CAD build for the part. Positions are in the model's coordinates, mm. Face numbers are marked on the shaded views. Give positions to 0.01 mm unless a question says otherwise; leave off trailing zeros.
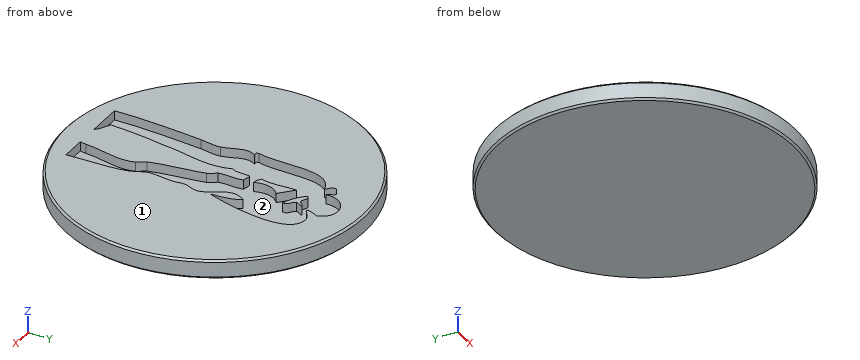
from build123d import *

# Parameters (mm, degrees)
POCKET_DEPTH = 1.25


with BuildPart() as part:
    # Sketch (on DatumPlane) → Revolution (revolve)
    with BuildSketch(Plane.YZ):
        Polygon((0, 0), (0, -2.5), (19.75, -2.5), (20, -2.25), (20, -0.25), (19.75, 0), align=None)
    revolve(axis=Axis((0, 0, 0), (0, 0, 1)))

    # Sketch005 (on DatumPlane) → Pocket (cut)
    with BuildSketch(Plane.XY):
        with BuildLine():
            add(Edge.make_bspline(
                [(2.212734, -16.79531), (2.353913, -15.955428)],
                knots=[0, 0, 11.60658, 11.60658], degree=1))
            add(Edge.make_bspline(
                [(2.353913, -15.955428), (2.452386, -13.484431), (3.666422, -11.326317), (2.913712, -8.958563)],
                knots=[0, 0, 0, 0, 1, 1, 1, 1], degree=3))
            add(Edge.make_bspline(
                [(2.913712, -8.958563), (2.776863, -8.528936), (2.33689, -8.25553), (2.213762, -7.839185)],
                knots=[0, 0, 0, 0, 1, 1, 1, 1], degree=3))
            add(Edge.make_bspline(
                [(2.213762, -7.839185), (1.63261, -5.878384), (1.420254, -2.638828), (0.954306, -0.562751)],
                knots=[0, 0, 0, 0, 1, 1, 1, 1], degree=3))
            add(Edge.make_bspline(
                [(0.954306, -0.562751), (0.837488, -0.042136), (0.287742, 0.418016), (0.254795, 0.556627)],
                knots=[0, 0, 0, 0, 1, 1, 1, 1], degree=3))
            add(Edge.make_bspline(
                [(0.254795, 0.556627), (0.035836, 1.475243), (0.405146, 2.931279), (0.114644, 3.915201)],
                knots=[0, 0, 0, 0, 1, 1, 1, 1], degree=3))
            add(Edge.make_bspline(
                [(0.114644, 3.915201), (-0.335749, 3.884236), (-0.477001, 4.162705), (-1.004588, 4.055279)],
                knots=[0, 0, 0, 0, 1, 1, 1, 1], degree=3))
            add(Edge.make_bspline(
                [(-1.004588, 4.055279), (-1.121992, 3.360832), (-0.906555, 2.162059), (-1.424455, 1.536367)],
                knots=[0, 0, 0, 0, 1, 1, 1, 1], degree=3))
            add(Edge.make_bspline(
                [(-1.424455, 1.536367), (-0.190168, -1.482321), (-1.911464, -5.34911), (-1.969652, -7.903684)],
                knots=[0, 0, 0, 0, 1, 1, 1, 1], degree=3))
            add(Edge.make_bspline(
                [(-1.969652, -7.903684), (-2.432446, -10.377469), (-2.703357, -13.113506), (-2.823623, -15.53644)],
                knots=[0, 0, 0, 0, 1, 1, 1, 1], degree=3))
            add(Edge.make_bspline(
                [(-2.823623, -15.53644), (-2.274023, -16.012809), (-1.385932, -16.150099), (-1.004588, -16.795897)],
                knots=[0, 0, 0, 0, 1, 1, 1, 1], degree=3))
            add(Edge.make_bspline(
                [(-1.004588, -16.795897), (-5.762036, -16.795897)],
                knots=[0, 0, 64.835, 64.835], degree=1))
            add(Edge.make_bspline(
                [(-5.762036, -16.795897), (-5.908571, -13.463225), (-5.538601, -8.73975), (-5.202677, -4.901359)],
                knots=[0, 0, 0, 0, 1, 1, 1, 1], degree=3))
            add(Edge.make_bspline(
                [(-5.202677, -4.901359), (-5.116898, -3.924994), (-4.784204, -3.058916), (-4.922814, -2.102804)],
                knots=[0, 0, 0, 0, 1, 1, 1, 1], degree=3))
            add(Edge.make_bspline(
                [(-4.922814, -2.102804), (-5.15799, -0.475138), (-6.392498, 0.658255), (-5.342242, 2.235731)],
                knots=[0, 0, 0, 0, 1, 1, 1, 1], degree=3))
            add(Edge.make_bspline(
                [(-5.342242, 2.235731), (-5.698637, 2.163087), (-5.885237, 1.997106), (-5.902261, 2.515373)],
                knots=[0, 0, 0, 0, 1, 1, 1, 1], degree=3))
            add(Edge.make_bspline(
                [(-5.902261, 2.515373), (-4.959136, 5.955324), (-6.879579, 11.869573), (-2.963554, 13.011331)],
                knots=[0, 0, 0, 0, 1, 1, 1, 1], degree=3))
            add(Edge.make_bspline(
                [(-2.963554, 13.011331), (-2.683178, 13.346374), (-3.817451, 13.457541), (-3.523427, 14.270347)],
                knots=[0, 0, 0, 0, 1, 1, 1, 1], degree=3))
            add(Edge.make_bspline(
                [(-3.523427, 14.270347), (-3.140321, 14.400739), (-2.926572, 14.699607), (-2.543613, 14.830292)],
                knots=[0, 0, 0, 0, 1, 1, 1, 1], degree=3))
            add(Edge.make_bspline(
                [(-2.543613, 14.830292), (-2.053816, 14.76051), (-2.204608, 14.0497), (-1.844029, 13.850773)],
                knots=[0, 0, 0, 0, 1, 1, 1, 1], degree=3))
            add(Edge.make_bspline(
                [(-1.844029, 13.850773), (-2.144071, 17.003889), (1.974624, 18.085918), (2.773854, 15.250087)],
                knots=[0, 0, 0, 0, 1, 1, 1, 1], degree=3))
            add(Edge.make_bspline(
                [(2.773854, 15.250087), (2.592685, 14.684491), (2.246708, 14.284215), (2.213762, 13.570469)],
                knots=[0, 0, 0, 0, 1, 1, 1, 1], degree=3))
            add(Edge.make_bspline(
                [(2.213762, 13.570469), (2.792786, 13.662925), (3.280014, 14.548962), (4.172728, 14.550283)],
                knots=[0, 0, 0, 0, 1, 1, 1, 1], degree=3))
            add(Edge.make_bspline(
                [(4.172728, 14.550283), (8.655083, 14.556593), (5.532639, 4.064598), (4.732674, 2.096606)],
                knots=[0, 0, 0, 0, 1, 1, 1, 1], degree=3))
            add(Edge.make_bspline(
                [(4.732674, 2.096606), (4.690702, 3.640108), (4.551504, 5.086751), (3.893159, 6.014246)],
                knots=[0, 0, 0, 0, 1, 1, 1, 1], degree=3))
            add(Edge.make_bspline(
                [(3.893159, 6.014246), (2.13422, 3.558659), (4.761805, 2.306173), (4.872605, 0.416989)],
                knots=[0, 0, 0, 0, 1, 1, 1, 1], degree=3))
            add(Edge.make_bspline(
                [(4.872605, 0.416989), (4.917146, -0.345406), (4.402694, -0.841587), (4.312953, -1.541977)],
                knots=[0, 0, 0, 0, 1, 1, 1, 1], degree=3))
            add(Edge.make_bspline(
                [(4.312953, -1.541977), (4.255498, -1.990169), (4.464992, -2.698558), (4.452811, -3.221668)],
                knots=[0, 0, 0, 0, 1, 1, 1, 1], degree=3))
            add(Edge.make_bspline(
                [(4.452811, -3.221668), (4.426028, -4.37979), (4.053783, -5.518319), (4.172802, -6.43943)],
                knots=[0, 0, 0, 0, 1, 1, 1, 1], degree=3))
            add(Edge.make_bspline(
                [(4.172802, -6.43943), (4.27487, -7.226994), (4.812289, -7.936631), (5.012317, -8.678994)],
                knots=[0, 0, 0, 0, 1, 1, 1, 1], degree=3))
            add(Edge.make_bspline(
                [(5.012317, -8.678994), (5.596477, -10.840703), (5.304801, -14.451403), (5.572409, -16.79531)],
                knots=[0, 0, 0, 0, 1, 1, 1, 1], degree=3))
            add(Edge.make_bspline(
                [(5.572409, -16.79531), (3.386852, -16.79531)],
                knots=[0, 0, 29.785, 29.785], degree=1))
            add(Edge.make_bspline(
                [(3.386852, -16.79531), (2.213542, -16.79531)],
                knots=[0, 0, 15.99, 15.99], degree=1))
            add(Edge.make_bspline(
                [(2.213542, -16.79531), (2.212734, -16.79531)],
                knots=[0, 0, 0.011, 0.011], degree=1))
        make_face()
        with BuildLine():
            add(Edge.make_bspline(
                [(0.814888, 12.031884), (0.306967, 12.149582), (-0.027122, 12.722883), (-0.444202, 12.172109)],
                knots=[0, 0, 0, 0, 1, 1, 1, 1], degree=3))
            add(Edge.make_bspline(
                [(-0.444202, 12.172109), (0.181271, 11.305297), (1.124615, 10.755404), (2.214129, 10.353001)],
                knots=[0, 0, 0, 0, 1, 1, 1, 1], degree=3))
            add(Edge.make_bspline(
                [(2.214129, 10.353001), (2.41379, 11.298327), (1.4408, 11.072396), (1.374613, 11.751948)],
                knots=[0, 0, 0, 0, 1, 1, 1, 1], degree=3))
            add(Edge.make_bspline(
                [(1.374613, 11.751948), (1.375934, 12.042671), (2.048515, 12.797141), (1.654256, 12.591903)],
                knots=[0, 0, 0, 0, 1, 1, 1, 1], degree=3))
            add(Edge.make_bspline(
                [(1.654256, 12.591903), (1.277828, 12.501942), (1.261465, 12.051476), (0.814888, 12.031884)],
                knots=[0, 0, 0, 0, 1, 1, 1, 1], degree=3))
        make_face(mode=Mode.SUBTRACT)
        with BuildLine():
            add(Edge.make_bspline(
                [(-1.144446, 5.595112), (-0.750334, 5.4758), (-0.569898, 5.143032), (-0.024554, 5.175244)],
                knots=[0, 0, 0, 0, 1, 1, 1, 1], degree=3))
            add(Edge.make_bspline(
                [(-0.024554, 5.175244), (-0.563587, 6.717205), (-0.133447, 7.929039), (0.814888, 8.67331)],
                knots=[0, 0, 0, 0, 1, 1, 1, 1], degree=3))
            add(Edge.make_bspline(
                [(0.814888, 8.67331), (0.225444, 9.250353), (-0.380877, 9.810005), (-1.004294, 10.352927)],
                knots=[0, 0, 0, 0, 1, 1, 1, 1], degree=3))
            add(Edge.make_bspline(
                [(-1.004294, 10.352927), (-1.116636, 8.904083), (-0.572319, 7.017394), (-1.144446, 5.595112)],
                knots=[0, 0, 0, 0, 1, 1, 1, 1], degree=3))
        make_face(mode=Mode.SUBTRACT)
    extrude(amount=-POCKET_DEPTH, mode=Mode.SUBTRACT)


solid = part.part
1. Wall check: line 1 (X direction, y = -12.5, z = -1.05); line 2 (X direction, y = -7.5, z = -0.5); line 3 (Y direction, x = 0.5, z = -0.9). Give the ranges that are in metal, low to high.
2. Pin check, flat tips, straight feed: P1, Ø1, axis at y = 0, z = -2, coming from the -X side; P2, Ø0.6, axis at x = 3.5, z = -0.5, coming from the +Y side; P3, Ø1, axis at y = -10, z = -0.5, coming from the -X side. Stop position of each tip, or through.
3. Mould opens along Y. For the marked faces 1 and 2 say: released by +Y, released by -Y, zero draft, split by the parting line, or undercut.
Reported:
1. line 1: x = -15.61 to -5.73, -2.6 to 2.94, 5.41 to 15.61
1. line 2: x = -18.54 to -5.42, -1.95 to 2.12, 4.52 to 18.54
1. line 3: y = -19.99 to 0.23, 8.39 to 8.98, 11.23 to 12.16, 16.88 to 19.99
2. P1: stops at x = -20
2. P2: stops at y = 19.74
2. P3: stops at x = -17.6
3. face 1: zero draft
3. face 2: undercut
